```python
from build123d import *

# Parameters (mm, degrees)
PAD_DEPTH       = 0.4
SKETCH001_R     = 2
POCKET_DEPTH    = 5
PAD001_DEPTH    = 6
POCKET001_DEPTH = 6.401
FILLET_R        = 0.5
FILLET001_R     = 0.39
FILLET002_R     = 0.9


with BuildPart() as part:
    # Sketch → Pad (new body)
    with BuildSketch(Plane.XY):
        with BuildLine():
            Line((-13.4, 6.275), (13.4, 6.275))
            ThreePointArc((15.4, 4.275), (14.814214, 5.689214), (13.4, 6.275))
            Line((15.4, 4.275), (15.4, -4.275))
            ThreePointArc((13.4, -6.275), (14.814214, -5.689214), (15.4, -4.275))
            Line((13.4, -6.275), (-13.4, -6.275))
            ThreePointArc((-15.4, -4.275), (-14.814214, -5.689214), (-13.4, -6.275))
            Line((-15.4, -4.275), (-15.4, 4.275))
            ThreePointArc((-13.4, 6.275), (-14.814214, 5.689214), (-15.4, 4.275))
        make_face()
    extrude(amount=PAD_DEPTH)

    # Sketch001 (on Face10 of Pad) → Pocket (cut)
    with BuildSketch(Plane.XY.offset(0.4)):
        with Locations((-12.495, 0)):
            Circle(SKETCH001_R)
        with Locations((12.495, 0)):
            Circle(SKETCH001_R)
    extrude(amount=-POCKET_DEPTH, mode=Mode.SUBTRACT)

    # Sketch002 (on Face5 of Pocket) → Pad001 (join)
    with BuildSketch(Plane.XY.offset(0.4)):
        with BuildLine():
            Line((-5.72, 4.6), (5.72, 4.6))
            ThreePointArc((8.674304, 1.078381), (8.018354, 3.5281), (5.72, 4.6))
            Line((8.674304, 1.078381), (8.109304, -2.121619))
            ThreePointArc((5.155, -4.6), (7.0831, -3.898354), (8.109304, -2.121619))
            Line((5.155, -4.6), (-5.155, -4.6))
            ThreePointArc((-8.109304, -2.121619), (-7.0831, -3.898354), (-5.155, -4.6))
            Line((-8.109304, -2.121619), (-8.674304, 1.078381))
            ThreePointArc((-5.72, 4.6), (-8.018354, 3.5281), (-8.674304, 1.078381))
        make_face()
    extrude(amount=PAD001_DEPTH)

    # Sketch003 (on Face21 of Pad001) → Pocket001 (cut, through all)
    with BuildSketch(Plane.XY.offset(6.4)):
        with BuildLine():
            Line((-5.72, 4.2), (5.72, 4.2))
            ThreePointArc((8.280397, 1.14793), (7.711906, 3.27102), (5.72, 4.2))
            Line((8.280397, 1.14793), (7.715397, -2.05207))
            ThreePointArc((5.155, -4.2), (6.82602, -3.591906), (7.715397, -2.05207))
            Line((5.155, -4.2), (-5.155, -4.2))
            ThreePointArc((-7.715397, -2.05207), (-6.82602, -3.591906), (-5.155, -4.2))
            Line((-7.715397, -2.05207), (-8.280397, 1.14793))
            ThreePointArc((-5.72, 4.2), (-7.711906, 3.27102), (-8.280397, 1.14793))
        make_face()
    extrude(amount=-POCKET001_DEPTH, mode=Mode.SUBTRACT)

    # Fillet
    fillet_edges = [part.edges().sort_by_distance(p)[0] for p in [
        (0, -4.6, 0.4),
    ]]
    fillet(fillet_edges, radius=FILLET_R)

    # Fillet001
    fillet001_edges = [part.edges().sort_by_distance(p)[0] for p in [
        (-7.0831, -3.898354, 6.4),
    ]]
    fillet(fillet001_edges, radius=FILLET001_R)

    # Fillet002
    fillet002_edges = [part.edges().sort_by_distance(p)[0] for p in [
        (0, 4.2, 0),
    ]]
    fillet(fillet002_edges, radius=FILLET002_R)


solid = part.part
```
Verification items for the finished model (mm, model axes). A direction names the side the tool comes from. Coordinates: 2 decimals unless noted, no trailing zeros. Loops run counter-clockwise (first coordinate to the right, second up) from the corner with the lowest first, then second, coordinate; pieces in that order, holes last. Notation, with made-up numbers: (85.5, -24.5) -> (121.5, -24.5) arc R22 ccw to (121.5, -18.5) -> close; hole circle Ø1 at (-37.75, 12.5). An arc over 180 degrees is marked (long way). Answer in a Markdown table with one row per item. Add a question column.
1. Section check B-B, the plane z = 4. Enter the section's corners in (x, y) (3 decimals), then the cut area to 3 significant figures.
2. Section check C-C, the plane y = 0. Give the number of separate pieces and of enclosed holes in the cut face, then the cut area to 3 significant figures.
3. Section check A-A, the plane x = -3. Enter the section's corners in (y, z) (3 decimals), then the cut area to 3 significant figures.
4. Draft check along X on faces 1 (the face through (7.06, -3.92, 3.42)), 2 (the face through (-8.39, -0.54, 3.42)), 3 (the face through (-6.845, -3.575, 3.689)). Enter one of: +X half, -X half, draft (parallel to the pull), parting line (faces both ways), or undercut.
5. Access from +Z, -Z, +X, -X, +Y, -Y to the whole of each face (thin tool, end or side, straight path). Record for faces 4 (the face through (0.07, -4.46, 0.27)), 5 (the face through (-8.544, -0.525, 0.543)), 6 (the face through (0, 4.6, 3)), 7 (the face through (0, -4.6, 3)), 8 (the face through (-7.994, -0.474, 3.689)).
6. Depth check by flat-ended pin: P1, Ø3.5, axis at x = 12.495, y = 0, coming from the +Z side; P2, Ø3, axis at x = -2, z = 4, coming from the +Y side; P3, Ø2, axis at y = -0.5, z = 5.5, coming from the +X side; P4, Ø2.5, axis at x = 1, z = 4.5, coming from the -Y side. Enter the tip coordinate at first touch or a pass-through.
7. Material ranges on probe 1 along Y at (x, z) = (-3, 2.5); probe 2 along Z at (x, y) = (-9, -5); probe 3 along X at (y, z) = (0.5, 4.75), recorded low to high. Write a range as [from, to].
Derived:
| question | item | result |
|---|---|---|
| 1 | outline | (-8.674, 1.078) -> (-8.109, -2.122) arc R3 ccw to (-5.155, -4.6) -> (5.155, -4.6) arc R3 ccw to (8.109, -2.122) -> (8.674, 1.078) arc R3 ccw to (5.72, 4.6) -> (-5.72, 4.6) arc R3 ccw to start; hole (-8.28, 1.148) -> (-7.715, -2.052) arc R2.6 ccw to (-5.155, -4.2) -> (5.155, -4.2) arc R2.6 ccw to (7.715, -2.052) -> (8.28, 1.148) arc R2.6 ccw to (5.72, 4.2) -> (-5.72, 4.2) arc R2.6 ccw to start |
| 1 | area | 18.3 mm² |
| 2 | separate pieces | 4 |
| 2 | enclosed holes | 0 |
| 2 | area | 7.22 mm² |
| 3 | outline | (-6.275, 0) -> (-5.1, 0) arc R0.9 ccw to (-4.2, 0.9) -> (-4.2, 6.4) -> (-4.21, 6.4) arc R0.39 ccw to (-4.6, 6.01) -> (-4.6, 0.9) arc R0.5 cw to (-5.1, 0.4) -> (-6.275, 0.4) -> close; (4.2, 0.9) arc R0.9 ccw to (5.1, 0) -> (6.275, 0) -> (6.275, 0.4) -> (5.1, 0.4) arc R0.5 cw to (4.6, 0.9) -> (4.6, 6.01) arc R0.39 ccw to (4.21, 6.4) -> (4.2, 6.4) -> close |
| 3 | area | 6.15 mm² |
| 4 | face 1 | +X half |
| 4 | face 2 | -X half |
| 4 | face 3 | undercut |
| 5 | face 4 | -Z |
| 5 | face 5 | +Z, -X, -Y |
| 5 | face 6 | +Z, +X, -X, +Y |
| 5 | face 7 | +Z, +X, -X, -Y |
| 5 | face 8 | +Z, -Z |
| 6 | P1 | passes through |
| 6 | P2 | stops at y = 4.6 |
| 6 | P3 | stops at x = 8.57 |
| 6 | P4 | stops at y = -4.6 |
| 7 | probe 1 | y = [-4.6, -4.2], [4.2, 4.6] |
| 7 | probe 2 | z = [0, 0.4] |
| 7 | probe 3 | x = [-8.57, -8.17], [8.17, 8.57] |
